Design review of the part built by this model. Coordinates are the model's own, in mm. Face numbers are marked on the shaded views. Round coordinates to 2 decimals unless told otherwise and drop trailing zeros. Order: outer loops, then holes, each group sorted by start corner. A loop starts at its lowest first (then second) coordinate and runs counter-clockwise, first axis right, second up. Notation, with made-up numbers: M 74.5,22 L 104.5,22 A18 ccw 104.5,53 Z; hole C -10.75,67.25 d8. An arc over 180 degrees is marked long. Write item = value, one per line. Start each with the question number.
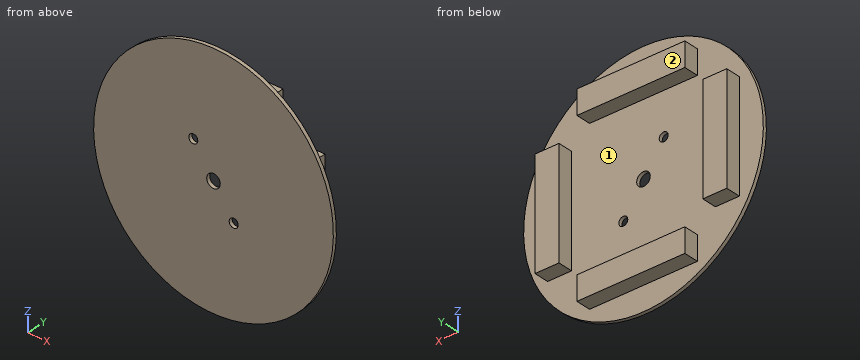
```python
from build123d import *

# Parameters (mm, degrees)
SKETCH1_R                    = 20
SKETCH1_R_2                  = 1.1303
SKETCH1_R_3                  = 0.75
PCB_DEPTH                    = 0.6
SKETCH2_W                    = 18
SKETCH2_H                    = 4
HIROSE_CONNECTOR_STACK_DEPTH = 2.5
CIRPATTERN1_COUNT            = 4


with BuildPart() as part:
    # Sketch1 → PCB (new body)
    with BuildSketch(Plane(origin=(0, 0, 0), x_dir=(1, 0, 0), z_dir=(0, 1, 0))):
        with Locations(Location((0, 0, 0), (0, 0, 270))):
            Circle(SKETCH1_R)
        with Locations(Location((0, 0, 0), (0, 0, 270))):
            Circle(SKETCH1_R_2, mode=Mode.SUBTRACT)
        with Locations(Location((3.372542584, 5, 0), (0, 0, 270))):
            Circle(SKETCH1_R_3, mode=Mode.SUBTRACT)
        with Locations(Location((-3.372542584, -5, 0), (0, 0, 270))):
            Circle(SKETCH1_R_3, mode=Mode.SUBTRACT)
    extrude(amount=PCB_DEPTH)

    # Sketch2 → Hirose Connector Stack (add)
    with BuildSketch(Plane(origin=(0, 0.6, 0), x_dir=(1, 0, 0), z_dir=(0, 1, 0))):
        with Locations((0, 14)):
            Rectangle(SKETCH2_W, SKETCH2_H)
    hirose_connector_stack = extrude(amount=HIROSE_CONNECTOR_STACK_DEPTH)

    # CirPattern1: Hirose Connector Stack ×4 about axis
    cirpattern1_axis = Axis((0, 0, 0), (0, 1, 0))
    for i in range(1, CIRPATTERN1_COUNT):
        add(hirose_connector_stack.rotate(cirpattern1_axis, i * 360 / CIRPATTERN1_COUNT))


solid = part.part
```
(1) Consider section D-D, the plane x = 12.5. Write out the cut boundary in (y, z).
(2) For line 1 along Z through (x, y) = (-3.5, 1.65); line 2 along X through (y, z) = (0.35, 0), list the stretches that pass through material, from the lowest coordinate up. Write a range as [from, to].
(3) Consider section B-B, the plane y = 1.9. Write out the cut boundary in (x, z).
(4) Draft analysis for pull direction X (two halves, no side actions). For the marked faces 1 and 2, state which applies: pulls with the +X half, pulls with the -X half, needs draft (parallel to the pull), parting line crosses it, or undercut.
(5) Insertion check: pin 1 (1.2 mm diameter, centred on y = 1.5, z = -14.5, fed in from +X); pin 2 (3.5 mm diameter, centred on x = 0, z = 0, fed in from +Y); pin 3 (0.8 mm diameter, centred on y = 1.5, z = 1.5, fed in from -X); pin 4 (1.2 mm diameter, centred on x = -3.37, z = 5, fed in from +Y) (1 decimal). Each pin has a flat end and moves straight along its axis. Give the tip position at first contact, or say it passes through.
(6) Consider section A-A, the plane x = 0. Write out the cut boundary in (y, z).
(7) Consider section C-C, the plane z = 0. Write out the cut boundary in (x, y).
Completed:
q1.outline = M 0,-15.61 L 0.6,-15.61 L 0.6,-9 L 3.1,-9 L 3.1,9 L 0.6,9 L 0.6,15.61 L 0,15.61 Z
q2.line_1 = [-16, -12], [12, 16]
q2.line_2 = [-20, -1.13], [1.13, 20]
q3.outline = M -16,-9 L -12,-9 L -12,9 L -16,9 Z; M -9,-16 L 9,-16 L 9,-12 L -9,-12 Z; M -9,12 L 9,12 L 9,16 L -9,16 Z; M 12,-9 L 16,-9 L 16,9 L 12,9 Z
q4.face_1 = undercut
q4.face_2 = needs draft
q5.pin_1 = 9
q5.pin_2 = 0.6
q5.pin_3 = -16
q5.pin_4 = through
q6.outline = M 0,-20 L 0.6,-20 L 0.6,-16 L 3.1,-16 L 3.1,-12 L 0.6,-12 L 0.6,-1.13 L 0,-1.13 Z; M 0,1.13 L 0.6,1.13 L 0.6,12 L 3.1,12 L 3.1,16 L 0.6,16 L 0.6,20 L 0,20 Z
q7.outline = M -20,0 L -1.13,0 L -1.13,0.6 L -12,0.6 L -12,3.1 L -16,3.1 L -16,0.6 L -20,0.6 Z; M 1.13,0 L 20,0 L 20,0.6 L 16,0.6 L 16,3.1 L 12,3.1 L 12,0.6 L 1.13,0.6 Z
